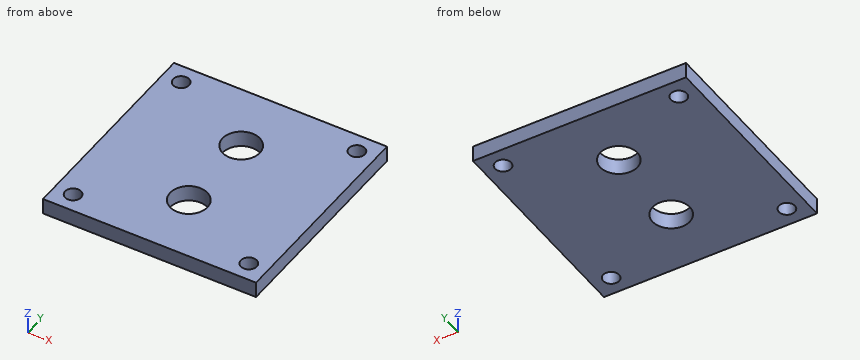
from build123d import *

# Parameters (mm, degrees)
SKETCH1_W           = 127
SKETCH1_H           = 127
BOSS_EXTRUDE1_DEPTH = 9.525
SKETCH2_R           = 11.1125
CUT_EXTRUDE1_DEPTH  = 9.525
SKETCH3_R           = 4.7625
CUT_EXTRUDE2_DEPTH  = 9.525


with BuildPart() as part:
    # Sketch1 → Boss-Extrude1 (new body)
    with BuildSketch(Plane.XY):
        Rectangle(SKETCH1_W, SKETCH1_H)
    extrude(amount=BOSS_EXTRUDE1_DEPTH)

    # Sketch2 → Cut-Extrude1 (cut)
    with BuildSketch(Plane(origin=(0, 0, 0), x_dir=(-1, 0, 0), z_dir=(0, 0, -1))):
        with Locations((0, 25.4)):
            Circle(SKETCH2_R)
        with Locations((0, -25.4)):
            Circle(SKETCH2_R)
    extrude(amount=-CUT_EXTRUDE1_DEPTH, mode=Mode.SUBTRACT)

    # Sketch3 → Cut-Extrude2 (cut)
    with BuildSketch(Plane(origin=(0, 0, 0), x_dir=(-1, 0, 0), z_dir=(0, 0, -1))):
        with Locations((52.3875, 52.3875)):
            Circle(SKETCH3_R)
        with Locations((52.3875, -52.3875)):
            Circle(SKETCH3_R)
        with Locations((-52.3875, 52.3875)):
            Circle(SKETCH3_R)
        with Locations((-52.3875, -52.3875)):
            Circle(SKETCH3_R)
    extrude(amount=-CUT_EXTRUDE2_DEPTH, mode=Mode.SUBTRACT)


solid = part.part
Model file for the job. Use its own axes, mm. Give positions to 0.01 mm unless a question says otherwise; leave off trailing zeros. Loops run counter-clockwise (first coordinate to the right, second up) from the corner with the lowest first, then second, coordinate; pieces in that order, holes last.
1) Wall check: line 1 (Y direction, x = 0, z = 4); line 2 (Y direction, x = 9.5, z = 7.5); line 3 (X direction, y = -15.5, z = 1). Give the ranges that are in metal, low to high.
2) Saw through at A-A (y = 25.4). Write the cut outline in (x, z) (1 decimal), plus the area to 3 significant figures.
3) Saw through at B-B (x = 0). Write the cut outline in (y, z) (1 decimal).
4) Saw through at D-D (y = -16). Write the cut outline in (x, z) (3 decimals).
5) Saw through at C-C (z = 2.5). Count the separate pieces of the cut face and the enclosed holes in it, plus the area to 3 significant figures.
Answer block:
1. line 1: y = -63.5 to -36.51, -14.29 to 14.29, 36.51 to 63.5
1. line 2: y = -63.5 to -31.17, -19.63 to 19.63, 31.17 to 63.5
1. line 3: x = -63.5 to -5.05, 5.05 to 63.5
2. outline: (-63.5, 0) - (-11.1, 0) - (-11.1, 9.5) - (-63.5, 9.5) - close; (11.1, 0) - (63.5, 0) - (63.5, 9.5) - (11.1, 9.5) - close
2. area: 998 mm2
3. outline: (-63.5, 0) - (-36.5, 0) - (-36.5, 9.5) - (-63.5, 9.5) - close; (-14.3, 0) - (14.3, 0) - (14.3, 9.5) - (-14.3, 9.5) - close; (36.5, 0) - (63.5, 0) - (63.5, 9.5) - (36.5, 9.5) - close
4. outline: (-63.5, 0) - (-5.927, 0) - (-5.927, 9.525) - (-63.5, 9.525) - close; (5.927, 0) - (63.5, 0) - (63.5, 9.525) - (5.927, 9.525) - close
5. separate pieces: 1
5. enclosed holes: 6
5. area: 15,100 mm2
